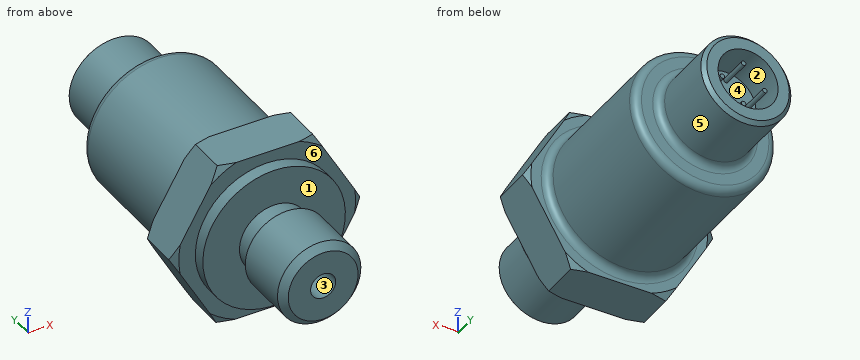
from build123d import *

# Parameters (mm, degrees)
SKETCH1_R               = 5.55625
EXTRUDE1_DEPTH          = 8.2
SKETCH2_R               = 4.6228
EXTRUDE2_DEPTH          = 2.9
SKETCH17_R              = 9.5
EXTRUDE13_DEPTH         = 1.7
EXTRUDE4_DEPTH          = 6
SKETCH5_R               = 9.5
EXTRUDE5_DEPTH          = 19.3
CHAMFER1_SIZE           = 0.9
FILLET1_R               = 1
SKETCH8_R               = 1.675
CUT_EXTRUDE1_DEPTH      = 4.9022
CUT_EXTRUDE1_DEPTH_BACK = 3.5
SKETCH14_R              = 6
EXTRUDE11_DEPTH         = 9.7
FILLET2_R               = 1
CHAMFER3_SIZE           = 0.5
SKETCH15_R              = 4
CUT_EXTRUDE2_DEPTH      = 5
SKETCH16_R              = 0.3
EXTRUDE12_DEPTH         = 4
CIRPATTERN1_COUNT       = 4


with BuildPart() as part:
    # Sketch1 → Extrude1 (new body)
    with BuildSketch(Plane(origin=(0, 0, 0), x_dir=(1, 0, 0), z_dir=(0, 1, 0))):
        with Locations(Location((0, 0, 0), (0, 0, 270))):  # turned: the seam where the file's is
            Circle(SKETCH1_R)
    extrude(amount=EXTRUDE1_DEPTH)

    # Sketch2 → Extrude2 (add)
    with BuildSketch(Plane(origin=(0, 8.2, 0), x_dir=(-1, 0, 0), z_dir=(0, 1, 0))):
        with Locations(Location((0, 0, 0), (0, 0, 90))):  # turned: the seam where the file's is
            Circle(SKETCH2_R)
    extrude(amount=EXTRUDE2_DEPTH)

    # Sketch17 → Extrude13 (add)
    with BuildSketch(Plane(origin=(0, 11.1, 0), x_dir=(-1, 0, 0), z_dir=(0, 1, 0))):
        with Locations(Location((0, 0, 0), (0, 0, 90))):  # turned: the seam where the file's is
            Circle(SKETCH17_R)
    extrude(amount=EXTRUDE13_DEPTH)

    # Sketch4 → Extrude4 (add)
    with BuildSketch(Plane(origin=(0, 12.8, 0), x_dir=(-1, 0, 0), z_dir=(0, 1, 0))):
        Polygon((12.701367758, 0.092684398), (6.270416836, 11.046049341), (-6.430950923, 10.953364943), (-12.701367758, -0.092684398), (-6.270416836, -11.046049341), (6.430950923, -10.953364943), align=None)
    extrude(amount=EXTRUDE4_DEPTH)

    # Sketch5 → Extrude5 (add)
    with BuildSketch(Plane(origin=(0, 18.8, 0), x_dir=(-1, 0, 0), z_dir=(0, 1, 0))):
        with Locations(Location((0, 0, 0), (0, 0, 90))):  # turned: the seam where the file's is
            Circle(SKETCH5_R)
    extrude(amount=EXTRUDE5_DEPTH)

    # Chamfer1
    chamfer1_edges = [part.edges().sort_by_distance(p)[0] for p in [
        (0, 0, -5.55625),
    ]]
    chamfer(chamfer1_edges, length=CHAMFER1_SIZE)

    # Fillet1
    fillet1_edges = [part.edges().sort_by_distance(p)[0] for p in [
        (0, 18.8, -9.5),
        (0, 38.1, -9.5),
    ]]
    fillet(fillet1_edges, radius=FILLET1_R)

    # Sketch7 → Cut-Revolve1 (revolve, cut)
    with BuildSketch(Plane.XY):
        Polygon((-12.701367758, 18.8), (-12.701367758, 18.222649731), (-11.701367758, 18.8), align=None)
        Polygon((-12.701367758, 12.8), (-12.701367758, 13.377350269), (-11.701367758, 12.8), align=None)
    revolve(axis=Axis((0.080267043, 18.8, 0), (0, -1, 0)), mode=Mode.SUBTRACT)

    # Sketch8 → Cut-Extrude1 (cut, two sides)
    with BuildSketch(Plane.XZ) as cut_extrude1_sk:
        with Locations(Location((0, 0, 0), (0, 0, 270))):  # turned: the seam where the file's is
            Circle(SKETCH8_R)
    extrude(amount=CUT_EXTRUDE1_DEPTH, mode=Mode.SUBTRACT)
    extrude(cut_extrude1_sk.sketch, amount=-CUT_EXTRUDE1_DEPTH_BACK, mode=Mode.SUBTRACT)

    # Sketch14 → Extrude11 (add)
    with BuildSketch(Plane(origin=(0, 38.1, 0), x_dir=(-1, 0, 0), z_dir=(0, 1, 0))):
        with Locations(Location((0, 0, 0), (0, 0, 90))):  # turned: the seam where the file's is
            Circle(SKETCH14_R)
    extrude(amount=EXTRUDE11_DEPTH)

    # Fillet2
    fillet2_edges = [part.edges().sort_by_distance(p)[0] for p in [
        (0, 38.1, -6),
    ]]
    fillet(fillet2_edges, radius=FILLET2_R)

    # Chamfer3
    chamfer3_edges = [part.edges().sort_by_distance(p)[0] for p in [
        (0, 47.8, -6),
    ]]
    chamfer(chamfer3_edges, length=CHAMFER3_SIZE)

    # Sketch15 → Cut-Extrude2 (cut)
    with BuildSketch(Plane(origin=(0, 47.8, 0), x_dir=(-1, 0, 0), z_dir=(0, 1, 0))):
        with Locations(Location((0, 0, 0), (0, 0, 90))):  # turned: the seam where the file's is
            Circle(SKETCH15_R)
    extrude(amount=-CUT_EXTRUDE2_DEPTH, mode=Mode.SUBTRACT)

    # Sketch16 → Extrude12 (add)
    with BuildSketch(Plane(origin=(0, 42.8, 0), x_dir=(-1, 0, 0), z_dir=(0, 1, 0))):
        with Locations(Location((0, -2.829193853, 0), (0, 0, 90))):  # turned: the seam where the file's is
            Circle(SKETCH16_R)
    extrude12 = extrude(amount=EXTRUDE12_DEPTH)

    # CirPattern1: Extrude12 ×4 about axis
    cirpattern1_axis = Axis((0, 0, 0), (0, -1, 0))
    for i in range(1, CIRPATTERN1_COUNT):
        add(extrude12.rotate(cirpattern1_axis, i * 360 / CIRPATTERN1_COUNT))


solid = part.part
For this review, take the finished solid that the model builds, in its own axes (mm). Face numbers are marked on the shaded views. A direction names the side the tool comes from. Round coordinates to 2 decimals unless told otherwise and drop trailing zeros. Loops run counter-clockwise (first coordinate to the right, second up) from the corner with the lowest first, then second, coordinate; pieces in that order, holes last. Notation, with made-up numbers: (75.25, 5.25) - (106.25, 5.25) arc R24 cw to (106.25, 40.25) - close; hole circle Ø4 at (17.5, 16.25). An arc over 180 degrees is marked (long way). Answer as CSV lines item,"result".
(1) Wall thickness on line 1 (X direction, y = 1.9, z = 0) (3 decimals); line 2 (Y direction, x = -5.25, z = -9); line 3 (Y direction, x = -7.75, z = -3): over which ranges is each line inside the solid? List them lowest first.
Checked values:
line 1,"x = -5.556 to -1.675, 1.675 to 5.556"
line 2,"y = 12.8 to 18.8"
line 3,"y = 11.1 to 38.1"
(2) Consider section A-A on y = 44.5. Give the boundary of the cut face in (x, z), then the cut area to 3 significant figures.
Checked values:
outline,"circle Ø12 at (0, 0); circle Ø0.6 at (-2.83, 0); circle Ø0.6 at (0, -2.83); circle Ø0.6 at (0, 2.83); circle Ø0.6 at (2.83, 0); hole circle Ø8 at (0, 0)"
area,"64.0 mm2"
(3) Tool access review of the marked faces 1, 2 and 3: name each direction out of +Z, -Z, +X, -X, +Y, -Y from which nothing blocks a thin tool from reaching the whole face with its end or side.
Checked values:
face 1,"none"
face 2,"+Y"
face 3,"-Y"
(4) Mouldability with a two-part tool opening along Z and no side actions: class the marked faces 4, 5 and 6 as +Z half, -Z half, draft (parallel to the pull), parting line (faces both ways), or undercut.
Checked values:
face 4,"undercut"
face 5,"parting line"
face 6,"draft"
(5) Insertion check: P1, Ø6, axis at x = 4.5, z = 4, coming from the -Y side; P2, Ø10, axis at x = 5, y = 27.5, coming from the -Z side; P3, Ø1, axis at y = 29.5, z = 5.5, coming from the +X side; P4, Ø4.5, axis at x = 0, z = 0, coming from the +Y side. Each pin has a flat end and moves straight along its axis. Give the tip position at first contact, or say it passes through.
Checked values:
P1,"stops at y = 0"
P2,"stops at z = -9.5"
P3,"stops at x = 8.08"
P4,"stops at y = 42.8"
(6) Consider section B-B on y = 12. Give the boundary of the cut face in (x, z).
Checked values:
outline,"circle Ø19 at (0, 0)"
